Source: three-view drawing plus pictorial views. Frame: mm from the lowest corner of the part. A direction names the side the tool comes from. Coordinates: 2 decimals unless noted, no trailing zeros. Loops run counter-clockwise (first coordinate to the right, second up) from the corner with the lowest first, then second, coordinate; pieces in that order, holes last. Notation, with made-up numbers: (78.5, 71.5) - (88.5, 71.5) arc R26 cw to (88.5, 107.5) - close; hole circle Ø8 at (51.25, 42.25). An arc over 180 degrees is marked (long way). Answer as CSV lines item,"result". Start each with the question number.
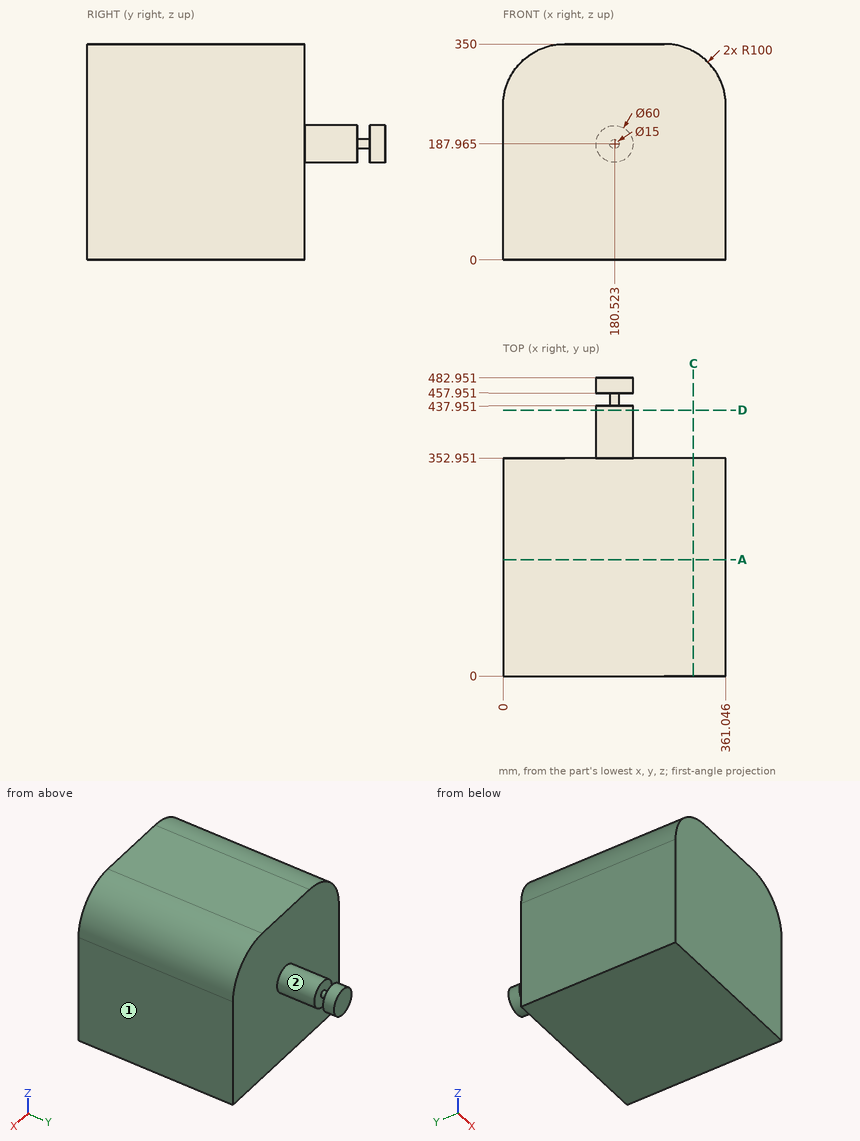
Item 1: Material intervals for probe 1 along Y at (x, z) = (321.5, 234.5); probe 2 along Z at (x, y) = (99.5, 158); probe 3 along Z at (x, y) = (158.5, 377) (1 decimal), sorted ascending.
Item 2: Section query A-A, the plane y = 188.5. Output: boundary loops of the cut face in (x, z) (1 decimal), and give its area (3 significant figures).
Item 3: Contact query for flat-ended pins moving along their axis: P1, Ø4, axis at y = 133, z = 239, coming from the -X side; P2, Ø8, axis at x = 45, z = 36, coming from the +Y side; P3, Ø5, axis at x = 300, y = 268.5, coming from the +Z side. Output: stop coordinate, or through.
Item 4: Section query D-D, the plane y = 431. Output: boundary loops of the cut face in (x, z) (1 decimal), and give its area (3 significant figures).
Item 5: Set-up query: the marked faces 1 and 2. Return all of +Z, -Z, +X, -X, +Y, -Y with unobstructed straight access to the full face (end or side cutting, diameter ignored); none if empty.
Item 6: Section query C-C, the plane x = 308.5. Output: boundary loops of the cut face in (y, z).
Response values:
1,probe 1,"y = 0 to 352.95"
1,probe 2,"z = 0 to 350"
1,probe 3,"z = 167.6 to 208.3"
2,outline,"(0, 0) - (361, 0) - (361, 250) arc R100 ccw to (261, 350) - (100, 350) arc R100 ccw to (0, 250) - close"
2,area,"122,000 mm²"
3,P1,"stops at x = 0"
3,P2,"stops at y = 352.95"
3,P3,"stops at z = 343.12"
4,outline,"circle Ø60 at (180.5, 188)"
4,area,"2,830 mm²"
5,face 1,"+Z, -Z, +X, +Y, -Y"
5,face 2,"+Y"
6,outline,"(0, 0) - (352.95, 0) - (352.95, 338.02) - (0, 338.02) - close"
